Build history of the part. All positions in model axes, mm. A direction names the side the tool comes from. Give positions to 0.01 mm unless a question says otherwise; leave off trailing zeros. Loops run counter-clockwise (first coordinate to the right, second up) from the corner with the lowest first, then second, coordinate; pieces in that order, holes last. Notation, with made-up numbers: M 65,-39.75 L 120,-39.75 A13 cw 120,-34.75 Z; hole C -21.5,79.5 d1. An arc over 180 degrees is marked long. Answer in a Markdown table with one row per item. Add a question column.
```python
from build123d import *

# Parameters (mm, degrees)
SKETCH_1_R          = 13.5
SKETCH_1_R_2        = 1.6
EXTRUDE_1_DEPTH     = 5
SKETCH_2_R          = 9
SKETCH_2_R_2        = 1.6
CUT_EXTRUDE_1_DEPTH = 150.490789026
CUT_EXTRUDE_2_DEPTH = 150.490789026
FILLET_1_R          = 2
FILLET_2_R          = 2
SKETCH_4_R          = 1.6
SKETCH_4_R_2        = 1.5
CUT_EXTRUDE_3_DEPTH = 150.490789026


with BuildPart() as part:
    # 草图1 → 凸台-拉伸1 (new body)
    with BuildSketch(Plane.XY):
        with BuildLine():
            Line((28, 0), (-28, 0))
            ThreePointArc((-28, 0), (-29.414213562, 0.585786438), (-30, 2))
            Line((-30, 2), (-30, 46.320508076))
            ThreePointArc((-30, 46.320508076), (-29.659258263, 48.908698527), (-28.660254038, 51.320508076))
            Line((-28.660254038, 51.320508076), (-11.132486541, 81.679491924))
            ThreePointArc((-11.132486541, 81.679491924), (-10.133482315, 84.091301473), (-9.792740578, 86.679491924))
            Line((-9.792740578, 86.679491924), (-9.792740578, 103.650604955))
            ThreePointArc((-9.792740578, 103.650604955), (-10.553945253, 107.477439278), (-12.721672766, 110.721672766))
            Line((-12.721672766, 110.721672766), (-15.071067812, 113.071067812))
            ThreePointArc((-15.071067812, 113.071067812), (-17.238795325, 116.3153013), (-18, 120.142135624))
            Line((-18, 120.142135624), (-18, 143))
            ThreePointArc((-18, 143), (-17.121320344, 145.121320344), (-15, 146))
            Line((-15, 146), (15, 146))
            ThreePointArc((15, 146), (17.121320344, 145.121320344), (18, 143))
            Line((18, 143), (18, 118.069065994))
            ThreePointArc((18, 118.069065994), (18.207415327, 116.0429156), (18.821057084, 114.100816135))
            Line((18.821057084, 114.100816135), (30.90426409, 86.151198222))
            ThreePointArc((30.90426409, 86.151198222), (31.567588607, 83.952064463), (31.711616521, 81.659588801))
            Line((31.711616521, 81.659588801), (30.013704652, 49.261500347))
            ThreePointArc((30.013704652, 49.261500347), (30.00342675, 48.999910267), (30, 48.738140784))
            Line((30, 48.738140784), (30, 2))
            ThreePointArc((30, 2), (29.414213562, 0.585786438), (28, 0))
        make_face()
        with Locations((0, 130)):
            Circle(SKETCH_1_R, mode=Mode.SUBTRACT)
        with Locations((-26, 11)):
            Circle(SKETCH_1_R_2, mode=Mode.SUBTRACT)
        with Locations((0, 4)):
            Circle(SKETCH_1_R_2, mode=Mode.SUBTRACT)
        with Locations((26, 11)):
            Circle(SKETCH_1_R_2, mode=Mode.SUBTRACT)
        with Locations((-13, 142)):
            Circle(SKETCH_1_R_2, mode=Mode.SUBTRACT)
        with Locations((13, 142)):
            Circle(SKETCH_1_R_2, mode=Mode.SUBTRACT)
        with Locations((13, 118)):
            Circle(SKETCH_1_R_2, mode=Mode.SUBTRACT)
        with Locations((-13, 118)):
            Circle(SKETCH_1_R_2, mode=Mode.SUBTRACT)
    extrude(amount=EXTRUDE_1_DEPTH)

    # 草图2 → 切除-拉伸1 (cut, through all)
    with BuildSketch(Plane.XY.offset(5)):
        with Locations((0, 40)):
            Circle(SKETCH_2_R)
        with Locations((-15, 48.5)):
            Circle(SKETCH_2_R_2)
        with Locations(Location((15, 48.5, 0), (0, 0, 180))):
            Circle(SKETCH_2_R_2)
        with Locations((15, 31.5)):
            Circle(SKETCH_2_R_2)
        with Locations(Location((-15, 31.5, 0), (0, 0, 180))):
            Circle(SKETCH_2_R_2)
    extrude(amount=-CUT_EXTRUDE_1_DEPTH, mode=Mode.SUBTRACT)

    # 草图3 → 切除-拉伸2 (cut, through all)
    with BuildSketch(Plane.XY.offset(5)):
        Polygon((-21, 23), (-21, 8), (-3, 8), align=None)
        Polygon((0, 9.405124838), (-21, 26.905124838), (21, 26.905124838), align=None)
        Polygon((21, 8), (3, 8), (21, 23), align=None)
        Polygon((-14.988893001, 59), (18.546418422, 59), (-1.565548778, 82.249914202), align=None)
        Polygon((22.739690965, 63.323631779), (23.875701286, 85), (3.988894601, 85), align=None)
        Polygon((-3.792740578, 111), (-3.792740578, 94.806657793), (10.309753882, 111), align=None)
        Polygon((-0.477589836, 91), (22.271324796, 91), (14.724663463, 108.45615222), align=None)
    extrude(amount=-CUT_EXTRUDE_2_DEPTH, mode=Mode.SUBTRACT)

    # 圆角1
    fillet_1_edges = [part.edges().sort_by_distance(p)[0] for p in [
        (21, 26.905124838, 2.5),
        (0, 9.405124838, 2.5),
        (-21, 26.905124838, 2.5),
        (21, 23, 2.5),
        (21, 8, 2.5),
        (3, 8, 2.5),
        (-21, 23, 2.5),
        (-3, 8, 2.5),
        (-21, 8, 2.5),
    ]]
    fillet(fillet_1_edges, radius=FILLET_1_R)

    # 圆角2
    fillet_2_edges = [part.edges().sort_by_distance(p)[0] for p in [
        (-3.792740578, 111, 2.5),
        (10.309753882, 111, 2.5),
        (-3.792740578, 94.806657793, 2.5),
        (14.724663463, 108.45615222, 2.5),
        (22.271324796, 91, 2.5),
        (-0.477589836, 91, 2.5),
        (-14.988893001, 59, 2.5),
        (-1.565548778, 82.249914202, 2.5),
        (18.546418422, 59, 2.5),
        (3.988894601, 85, 2.5),
        (23.875701286, 85, 2.5),
        (22.739690965, 63.323631779, 2.5),
    ]]
    fillet(fillet_2_edges, radius=FILLET_2_R)

    # 草图4 → 切除-拉伸3 (cut, through all)
    with BuildSketch(Plane.XY.offset(5)):
        with Locations((25.993043669, 49.095132548)):
            Circle(SKETCH_4_R)
        with Locations((28.171937238, 74)):
            Circle(SKETCH_4_R)
        with Locations((-19.196152423, 59.712812921)):
            Circle(SKETCH_4_R_2)
        with Locations((-15.196152423, 66.641016151)):
            Circle(SKETCH_4_R_2)
    extrude(amount=-CUT_EXTRUDE_3_DEPTH, mode=Mode.SUBTRACT)


solid = part.part
```
(1) Pull direction Y, two halves, no side cores. Call faces 1 (the flat face through (18, 131, 2)), 2 (the cylindrical face through (17.1, 145.14, 2.46)), 3 (the cylindrical face through (7.7, 109.9, 2.5)): +Y half, -Y half, draft (parallel to the pull), parting line (faces both ways), or undercut.
(2) Slice it at C-C, the plane z = 1.25. State how many separate pieces and enclosed holes the cut face has, then the cut area to 3 significant figures.
(3) Wall check: line 1 (X direction, y = 12, z = 0.8); line 2 (Y direction, x = -4, z = 4.05); line 3 (X direction, y = 60.5, z = 1.75). Give the ranges that are in metal, low to high.
(4) Slice it at B-B, the plane y = 130. Give the cut face in (x, z).
(5) Tool access for faces 4 (the cylindrical face through (-17.345, 25.618, 2.465)), 5 (the cylindrical face through (18.2, 116.07, 2.46)), 6 (the flat face through (30, 26, 2)): list every direction of +Z, -Z, +X, -X, +Y, -Y with a clear straight run to the whole face (end or side of a thin tool).
(6) Slice it at A-A, the plane y = 4. Give the cut face in (x, z).
Solution:
| question | item | result |
|---|---|---|
| 1 | face 1 | draft |
| 1 | face 2 | +Y half |
| 1 | face 3 | undercut |
| 2 | separate pieces | 1 |
| 2 | enclosed holes | 24 |
| 2 | area | 4,510 mm^2 |
| 3 | line 1 | -30 to -27.25, -24.75 to -21, -7.8 to -3.11, 3.11 to 7.8, 21 to 24.75, 27.25 to 30 |
| 3 | line 2 | 0 to 12.74, 26.91 to 31.94, 48.06 to 59, 78.03 to 117.11, 142.89 to 146 |
| 3 | line 3 | -23.36 to -20.47, -17.92 to -13.46, 16.11 to 30.6 |
| 4 | outline | M -18,0 L -13.5,0 L -13.5,5 L -18,5 Z; M 13.5,0 L 18,0 L 18,5 L 13.5,5 Z |
| 5 | face 4 | +Z, -Z |
| 5 | face 5 | +Z, -Z, +X, +Y |
| 5 | face 6 | +Z, -Z, +X, -Y |
| 6 | outline | M -30,0 L -1.6,0 L -1.6,5 L -30,5 Z; M 1.6,0 L 30,0 L 30,5 L 1.6,5 Z |
